Check sheet for the modelled part. Datum: model origin and axes. Units: mm. Face numbers are marked on the shaded views. A direction names the side the tool comes from. Give positions to 0.01 mm unless a question says otherwise; leave off trailing zeros. Order: outer loops, then holes, each group sorted by start corner. A loop starts at its lowest first (then second) coordinate and runs counter-clockwise, first axis right, second up.
Item 1: Gauge pin test, flat ends, axial feed: P1, Ø1.5, axis at x = -7.5, z = 18.5, coming from the +Y side; P2, Ø12, axis at y = 63, z = 14, coming from the +X side; P3, Ø1.5, axis at y = 17, z = 26, coming from the +X side. Record the tip position at first contact, or that the pin passes through.
Item 2: Release check for a two-part mould opening along X. For the marked faces 1, 2, 3 and 4 record: released by +X, released by -X, zero draft, split by the parting line, or undercut.
Item 3: Sectioned sample at A-A on x = 0. Record the boundary of the cut face in (y, z) (1 decimal).
Item 4: Sectioned sample at C-C on z = 4.5. Count the separate pieces of the cut face and the enclosed holes in it, and give its area (3 significant figures).
Item 5: Sectioned sample at B-B on y = 0. Record the boundary of the cut face in (x, z) (1 decimal).
Item 6: Material ranges on line 1 along Y through (x, z) = (0, 10) (1 decimal); line 2 along Y through (x, z) = (0, 19) (1 decimal); line 3 along X through (y, z) = (0, 11.5) (1 decimal), recorded low to high.
Item 7: Access from +Z, -Z, +X, -X, +Y, -Y to the whole of each face (thin tool, end or side, straight path). Record for the marked faces 5 and 6.
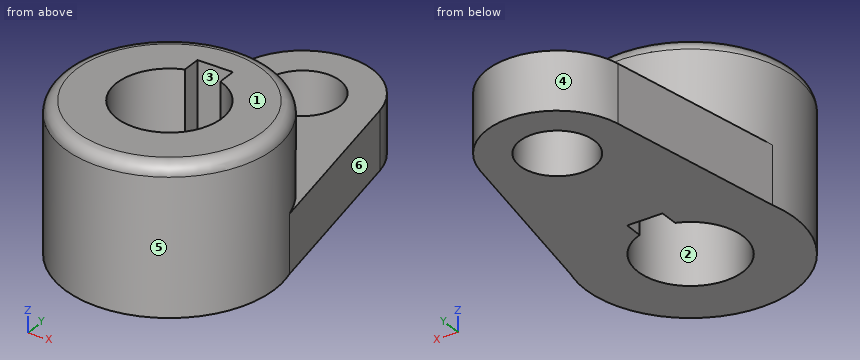
from build123d import *

# Parameters (mm, degrees)
F0_R     = 28.575
F0_R_2   = 14.2875
F1_DEPTH = 40.2336
F2_W     = 9.652
F2_H     = 5.081535
F3_DEPTH = 40.2346
F4_R     = 10.16
F5_DEPTH = 15.7734
F6_R     = 3.302


with BuildPart() as f1:
    # F0 (on Top) → F1 (new body)
    with BuildSketch(Plane.XY):
        Circle(F0_R)
        Circle(F0_R_2, mode=Mode.SUBTRACT)
    extrude(amount=F1_DEPTH)

    # F2 (on face) → F3 (cut, through all)
    with BuildSketch(Plane.XY.offset(40.2336)):
        with Locations((0, 15.988532)):
            Rectangle(F2_W, F2_H)
    extrude(amount=-F3_DEPTH, mode=Mode.SUBTRACT)

    # F4 (on Top) → F5 (join)
    with BuildSketch(Plane.XY):
        with BuildLine():
            ThreePointArc((18.760191, 57.285248), (0, 73.025), (-18.760191, 57.285248))
            Line((-18.760191, 57.285248), (-27.641075, 6.954561))
            ThreePointArc((-27.641075, 6.954561), (0, 28.502543), (27.641075, 6.954561))
            Line((27.641075, 6.954561), (18.760191, 57.285248))
        make_face()
        with Locations((0, 53.975)):
            Circle(F4_R, mode=Mode.SUBTRACT)
    extrude(amount=F5_DEPTH)

    # F6
    f6_edges = [f1.edges().sort_by_distance(p)[0] for p in [
        (-28.575, 0, 40.2336),
    ]]
    fillet(f6_edges, radius=F6_R)


solid = f1.part
Report:
1. P1: stops at y = 27.77
1. P2: stops at x = 18.81
1. P3: stops at x = 23.5
2. face 1: zero draft
2. face 2: undercut
2. face 3: undercut
2. face 4: split by the parting line
3. outline: (-28.6, 0) - (-14.3, 0) - (-14.3, 40.2) - (-25.3, 40.2) arc R3.3 ccw to (-28.6, 36.9) - close; (18.5, 0) - (43.8, 0) - (43.8, 15.8) - (28.6, 15.8) - (28.6, 36.9) arc R3.3 ccw to (25.3, 40.2) - (18.5, 40.2) - close; (64.1, 0) - (73, 0) - (73, 15.8) - (64.1, 15.8) - close
4. separate pieces: 1
4. enclosed holes: 2
4. area: 3,450 mm2
5. outline: (-28.6, 0) - (-14.3, 0) - (-14.3, 40.2) - (-25.3, 40.2) arc R3.3 ccw to (-28.6, 36.9) - close; (14.3, 0) - (28.6, 0) - (28.6, 36.9) arc R3.3 ccw to (25.3, 40.2) - (14.3, 40.2) - close
6. line 1: y = -28.6 to -14.3, 18.5 to 43.8, 64.1 to 73
6. line 2: y = -28.6 to -14.3, 18.5 to 28.6
6. line 3: x = -28.6 to -14.3, 14.3 to 28.6
7. face 5: +Z
7. face 6: +Z, -Z, +X, +Y
